```python
from build123d import *

# Parameters (mm, degrees)
SKETCH1_R           = 1.5
BOSS_EXTRUDE1_DEPTH = 3
FILLET1_R           = 1
FILLET2_R           = 3


with BuildPart() as part:
    # Sketch1 → Boss-Extrude1 (new body)
    with BuildSketch(Plane.XY):
        Polygon((6.25, 17.5), (8, 17.5), (8, 22.5), (-8, 22.5), (-8, 17.5), (-6.25, 17.5), (-6.25, -17.5), (6.25, -17.5), align=None)
        with Locations((0, 3.5)):
            Circle(SKETCH1_R, mode=Mode.SUBTRACT)
        with Locations((0, -12.5)):
            Circle(SKETCH1_R, mode=Mode.SUBTRACT)
    extrude(amount=BOSS_EXTRUDE1_DEPTH)

    # Fillet1
    fillet1_edges = [part.edges().sort_by_distance(p)[0] for p in [
        (6.25, 17.5, 1.5),
        (-6.25, 17.5, 1.5),
        (-8, 22.5, 1.5),
        (8, 22.5, 1.5),
    ]]
    fillet(fillet1_edges, radius=FILLET1_R)

    # Fillet2
    fillet2_edges = [part.edges().sort_by_distance(p)[0] for p in [
        (6.25, -17.5, 1.5),
        (-6.25, -17.5, 1.5),
    ]]
    fillet(fillet2_edges, radius=FILLET2_R)


solid = part.part
```
Verification items for the finished model (mm, model axes). A direction names the side the tool comes from. Coordinates: 2 decimals unless noted, no trailing zeros. Write each loop counter-clockwise with the first axis right and the second up, starting at its lowest first coordinate (ties: lowest second). Pieces come first, ordered by that corner, then holes. Notation, with made-up numbers: (42, 79.25) - (88, 79.25) arc R19 cw to (88, 105.25) - close; hole circle Ø3 at (77.25, 83.25). An arc over 180 degrees is marked (long way). One line per question, with ' | ' between items. Start each with the question number.
1. Section check A-A (y = 3.5). Enter the section's corners in (x, z), plus the area to 3 significant figures.
2. Section check C-C (z = 0.85). Enter the section's corners in (x, y).
3. Gauge pin test, flat end, axial feed: P1, Ø0.8, axis at x = 7.5, z = 2, coming from the -Y side. Record the tip position at first contact, or that the pin passes through.
4. Section check D-D (x = -5.5). Enter the section's corners in (y, z), plus the area to 3 significant figures.
5. Material ranges on line 1 along Y through (x, z) = (0, 1.9); line 2 along X through (y, z) = (-2, 0.4), recorded low to high.
6. Section check B-B (x = 0). Enter the section's corners in (y, z), plus the area to 3 significant figures.
7. Access from +Z, -Z, +X, -X, +Y, -Y to the whole of each face (thin tool, end or side, straight path). Record for faces 5 (the flat face through (8, 19, 1)), 6 (the flat face through (6.25, 1, 1)), 7 (the flat face through (-6.25, 1, 1)).
8. Draft check along X on faces 1 (the cylindrical face through (-6.535, 17.199, 1.521)), 2 (the flat face through (0, 22.5, 1)), 3 (the cylindrical face through (0, -14, 1)), 4 (the cylindrical face through (-1.5, 3.57, 1.48)). Enter one of: released by +X, released by -X, zero draft, split by the parting line, or undercut.
Computed values:
1) outline: (-6.25, 0) - (-1.5, 0) - (-1.5, 3) - (-6.25, 3) - close; (1.5, 0) - (6.25, 0) - (6.25, 3) - (1.5, 3) - close | area: 28.5 mm²
2) outline: (-8, 17.5) - (-7.25, 17.5) arc R1 cw to (-6.25, 16.5) - (-6.25, -14.5) arc R3 ccw to (-3.25, -17.5) - (3.25, -17.5) arc R3 ccw to (6.25, -14.5) - (6.25, 16.5) arc R1 cw to (7.25, 17.5) - (8, 17.5) - (8, 21.5) arc R1 ccw to (7, 22.5) - (-7, 22.5) arc R1 ccw to (-8, 21.5) - close; hole circle Ø3 at (0, -12.5); hole circle Ø3 at (0, 3.5)
3) P1: y = 17.49
4) outline: (-16.48, 0) - (22.5, 0) - (22.5, 3) - (-16.48, 3) - close | area: 117 mm²
5) line 1: -17.5 to -14, -11 to 2, 5 to 22.5 | line 2: -6.25 to 6.25
6) outline: (-17.5, 0) - (-14, 0) - (-14, 3) - (-17.5, 3) - close; (-11, 0) - (2, 0) - (2, 3) - (-11, 3) - close; (5, 0) - (22.5, 0) - (22.5, 3) - (5, 3) - close | area: 102 mm²
7) face 5: +Z, -Z, +X, +Y, -Y | face 6: +Z, -Z, +X, -Y | face 7: +Z, -Z, -X, -Y
8) face 1: released by -X | face 2: zero draft | face 3: undercut | face 4: undercut
